The listing builds one solid part. Answer for the finished solid, in the listing's coordinates (mm). Coordinates: 2 decimals unless noted, no trailing zeros. Write each loop counter-clockwise with the first axis right and the second up, starting at its lowest first coordinate (ties: lowest second). Pieces come first, ordered by that corner, then holes.
from build123d import *

# Parameters (mm, degrees)
SKETCH2_R           = 1.65
SKETCH2_R_2         = 11
SKETCH2_R_3         = 2.25
BOSS_EXTRUDE1_DEPTH = 3.8


with BuildPart() as part:
    # Sketch2 → Boss-Extrude1 (new body)
    with BuildSketch(Plane.XY):
        with BuildLine():
            Line((-170.5, 150), (-137.4, 150))
            ThreePointArc((-137.4, 150), (-135.985786438, 149.414213562), (-135.4, 148))
            Line((-135.4, 148), (-135.4, 25))
            Line((-135.4, 25), (135.4, 25))
            Line((135.4, 25), (135.4, 148))
            ThreePointArc((135.4, 148), (135.985786438, 149.414213562), (137.4, 150))
            Line((137.4, 150), (170.5, 150))
            ThreePointArc((170.5, 150), (171.914213562, 149.414213562), (172.5, 148))
            Line((172.5, 148), (172.5, 15.719548835))
            Line((172.5, 15.719548835), (162.5, 15.719548835))
            Line((162.5, 15.719548835), (162.5, -69.888900965))
            Line((162.5, -69.888900965), (172.5, -69.888900965))
            Line((172.5, -69.888900965), (172.5, -99))
            ThreePointArc((172.5, -99), (172.207106781, -99.707106781), (171.5, -100))
            Line((171.5, -100), (-169.5, -100))
            ThreePointArc((-169.5, -100), (-171.621320344, -99.121320344), (-172.5, -97))
            Line((-172.5, -97), (-172.5, -69.888900965))
            Line((-172.5, -69.888900965), (-162.5, -69.888900965))
            Line((-162.5, -69.888900965), (-162.5, 15.719548835))
            Line((-162.5, 15.719548835), (-172.5, 15.719548835))
            Line((-172.5, 15.719548835), (-172.5, 148))
            ThreePointArc((-172.5, 148), (-171.914213562, 149.414213562), (-170.5, 150))
        make_face()
        with Locations(Location((-168.334802826, 116, 0), (0, 0, 180))):
            Circle(SKETCH2_R, mode=Mode.SUBTRACT)
        with Locations(Location((-139.665197174, 116, 0), (0, 0, 180))):
            Circle(SKETCH2_R, mode=Mode.SUBTRACT)
        with Locations(Location((168.334802826, 116, 0), (0, 0, 180))):
            Circle(SKETCH2_R, mode=Mode.SUBTRACT)
        with Locations(Location((139.665197174, 116, 0), (0, 0, 180))):
            Circle(SKETCH2_R, mode=Mode.SUBTRACT)
        with Locations(Location((154, 116, 0), (0, 0, 180))):
            Circle(SKETCH2_R_2, mode=Mode.SUBTRACT)
        with Locations(Location((-154, 116, 0), (0, 0, 180))):
            Circle(SKETCH2_R_2, mode=Mode.SUBTRACT)
        with Locations(Location((152.5, -52.584676065, 0), (0, 0, 180))):
            Circle(SKETCH2_R, mode=Mode.SUBTRACT)
        with Locations(Location((152.5, -1.584676065, 0), (0, 0, 180))):
            Circle(SKETCH2_R, mode=Mode.SUBTRACT)
        with Locations(Location((-152.5, -52.584676065, 0), (0, 0, 180))):
            Circle(SKETCH2_R, mode=Mode.SUBTRACT)
        with Locations(Location((-152.5, -1.584676065, 0), (0, 0, 180))):
            Circle(SKETCH2_R, mode=Mode.SUBTRACT)
        with Locations(Location((-30, -42.029676065, 0), (0, 0, 180))):
            Circle(SKETCH2_R_3, mode=Mode.SUBTRACT)
        with Locations(Location((-30, -12.139676065, 0), (0, 0, 180))):
            Circle(SKETCH2_R_3, mode=Mode.SUBTRACT)
        with Locations(Location((-54.06, -12.139676065, 0), (0, 0, 180))):
            Circle(SKETCH2_R_3, mode=Mode.SUBTRACT)
        with Locations(Location((-54.06, -42.029676065, 0), (0, 0, 180))):
            Circle(SKETCH2_R_3, mode=Mode.SUBTRACT)
        with Locations(Location((54.06, -42.029676065, 0), (0, 0, 180))):
            Circle(SKETCH2_R_3, mode=Mode.SUBTRACT)
        with Locations(Location((30, -42.029676065, 0), (0, 0, 180))):
            Circle(SKETCH2_R_3, mode=Mode.SUBTRACT)
        with Locations(Location((30, -12.139676065, 0), (0, 0, 180))):
            Circle(SKETCH2_R_3, mode=Mode.SUBTRACT)
        with Locations(Location((54.06, -12.139676065, 0), (0, 0, 180))):
            Circle(SKETCH2_R_3, mode=Mode.SUBTRACT)
        with Locations(Location((-123.526576723, -81.066130201, 0), (0, 0, 180))):
            Circle(SKETCH2_R, mode=Mode.SUBTRACT)
        with Locations(Location((-152.186576723, -81.066130201, 0), (0, 0, 180))):
            Circle(SKETCH2_R, mode=Mode.SUBTRACT)
        with Locations(Location((-137.856576723, -81.066130201, 0), (0, 0, 180))):
            Circle(SKETCH2_R_2, mode=Mode.SUBTRACT)
        with Locations(Location((123.526576723, -81.066130201, 0), (0, 0, 180))):
            Circle(SKETCH2_R, mode=Mode.SUBTRACT)
        with Locations(Location((152.186576723, -81.066130201, 0), (0, 0, 180))):
            Circle(SKETCH2_R, mode=Mode.SUBTRACT)
        with Locations(Location((137.856576723, -81.066130201, 0), (0, 0, 180))):
            Circle(SKETCH2_R_2, mode=Mode.SUBTRACT)
        with BuildLine():
            Line((-67.457425662, 10.086727014), (-113.055173681, 10.086727014))
            ThreePointArc((-113.055173681, 10.086727014), (-115.883600806, 8.915154139), (-117.055173681, 6.086727014))
            Line((-117.055173681, 6.086727014), (-117.055173681, -60.256079145))
            ThreePointArc((-117.055173681, -60.256079145), (-115.883600806, -63.084506269), (-113.055173681, -64.256079145))
            Line((-113.055173681, -64.256079145), (-67.457425662, -64.256079145))
            ThreePointArc((-67.457425662, -64.256079145), (-64.628998537, -63.084506269), (-63.457425662, -60.256079145))
            Line((-63.457425662, -60.256079145), (-63.457425662, 6.086727014))
            ThreePointArc((-63.457425662, 6.086727014), (-64.628998537, 8.915154139), (-67.457425662, 10.086727014))
        make_face(mode=Mode.SUBTRACT)
        with BuildLine():
            Line((67.457425662, 10.086727014), (113.055173681, 10.086727014))
            ThreePointArc((113.055173681, 10.086727014), (115.883600806, 8.915154139), (117.055173681, 6.086727014))
            Line((117.055173681, 6.086727014), (117.055173681, -60.256079145))
            ThreePointArc((117.055173681, -60.256079145), (115.883600806, -63.084506269), (113.055173681, -64.256079145))
            Line((113.055173681, -64.256079145), (67.457425662, -64.256079145))
            ThreePointArc((67.457425662, -64.256079145), (64.628998537, -63.084506269), (63.457425662, -60.256079145))
            Line((63.457425662, -60.256079145), (63.457425662, 6.086727014))
            ThreePointArc((63.457425662, 6.086727014), (64.628998537, 8.915154139), (67.457425662, 10.086727014))
        make_face(mode=Mode.SUBTRACT)
    extrude(amount=BOSS_EXTRUDE1_DEPTH)


solid = part.part
1. Section A-A on y = 66.5 is taken. Give the vertices of the cut face in (x, z).
Results found:
outline: (-172.5, 0) - (-135.4, 0) - (-135.4, 3.8) - (-172.5, 3.8) - close; (135.4, 0) - (172.5, 0) - (172.5, 3.8) - (135.4, 3.8) - close
2. Section C-C on z = 0.9 is taken. State how many separate pieces and enclosed holes the cut face has, then the cut area to 3 significant figures.
Results found:
separate pieces: 1
enclosed holes: 26
area: 41,000 mm2
3. Section B-B on x = 15.5 is taken. Give the vertices of the cut face in (y, z), then the cut area to 3 significant figures.
Results found:
outline: (-100, 0) - (25, 0) - (25, 3.8) - (-100, 3.8) - close
area: 475 mm2
4. Find the intervals of material crossed by L1, parallel to Y at x = 54.06, z = 1.2; L2, parallel to X at y = -17.5, z = 0.65; L3, parallel to X at y = 37, z = 1.95, in increasing order.
Results found:
L1: y = -100 to -44.28, -39.78 to -14.39, -9.89 to 25
L2: x = -162.5 to -117.06, -63.46 to 63.46, 117.06 to 162.5
L3: x = -172.5 to -135.4, 135.4 to 172.5
5. For a pull along Y with two mould halves and no side action, classify faces 1 (the cylindrical face through (165, 116, 2)), 2 (the flat face through (2, -29, 0)), 3 (the cylindrical face through (127.365, -84.37, 1.873)) as pulls with the +Y half, pulls with the -Y half, needs draft (parallel to the pull), parting line crosses it, or undercut.
Results found:
face 1: undercut
face 2: needs draft
face 3: undercut
6. Flat-ended cylindrical pins translate along their axes: P1, Ø2, axis at x = -152.19, y = -81.07, coming from the -Z side (3 decimals); P2, Ø1.1, axis at y = -16, z = 3, coming from the +X side; P3, Ø1.9, axis at y = -12.5, z = 2.5, coming from the -X side. Find the tip coordinate at first contact, or state that the pin passes through.
Results found:
P1: passes through
P2: stops at x = 162.5
P3: stops at x = -162.5
